Build history of the part. All positions in model axes, mm. A direction names the side the tool comes from. Give positions to 0.01 mm unless a question says otherwise; leave off trailing zeros. Write each loop counter-clockwise with the first axis right and the second up, starting at its lowest first coordinate (ties: lowest second). Pieces come first, ordered by that corner, then holes. Notation, with made-up numbers: (86, 6) -> (144, 6) arc R36 ccw to (144, 40) -> close; hole circle Ø11 at (5.5, 67). An arc over 180 degrees is marked (long way). Write item = value, one per line. Start each with the question number.
Q1. Wall check: line 1 (Y direction, x = 9.25, z = 0); line 2 (X direction, y = -1.5, z = -13); line 3 (Z direction, x = 1.5, y = 2). Give the ranges that are in metal, low to high.
Q2. Saw through at C-C, the plane x = 2.5. List the corners of the cut face in (y, z), then the cut area to 3 significant figures.
Q3. Mould opens along Y. For faces 1 (the face through (2.03, -3.47, 15.62)), 2 (the face through (15, 0, 3)), 3 (the face through (7.4, -2.26, 1.18)) say: pulls with the +Y half, pulls with the -Y half, needs draft (parallel to the pull), parting line crosses it, or undercut.
Q4. Tool access for faces 4 (the face through (0, 0, 3)), 5 (the face through (4, -10, 8)): list every direction of +Z, -Z, +X, -X, +Y, -Y with a clear straight run to the whole face (end or side of a thin tool).
Q5. Drop flat-ended pins along their axis: P1, Ø4, axis at x = 8, y = -4.5, coming from the -Z side; P2, Ø1.5, axis at x = 5, z = 3, coming from the -Y side; P3, Ø2, axis at y = 4.5, z = -2, coming from the -X side; P4, Ø2, axis at x = 4.5, z = -7, coming from the +Y side. Give the stop position or say it passes through.
Q6. Saw through at D-D, the plane y = -11. List the corners of the cut face in (x, z).
Q7. Saw through at A-A, the plane y = 0. List the corners of the cut face in (x, z), then the cut area to 4 significant figures.
from build123d import *

# Parameters (mm, degrees)
SKETCH2_R          = 2.55
CUT_EXTRUDE1_DEPTH = 15


with BuildPart() as part:
    # Sketch1 → Revolve1 (revolve)
    with BuildSketch(Plane.XY):
        Polygon((0, 0), (0, 16), (4, 16), (4, 12.5), (11, 12.5), (11, 16), (15, 16), (15, 0), align=None)
    revolve(axis=Axis((15, 0, 0), (-1, 0, 0)))

    # Sketch2 → Cut-Extrude1 (cut)
    with BuildSketch(Plane.ZY):
        Circle(SKETCH2_R)
    extrude(amount=-CUT_EXTRUDE1_DEPTH, mode=Mode.SUBTRACT)


solid = part.part
Report:
q1.line_1 = -12.5 to -2.55, 2.55 to 12.5
q1.line_2 = 0 to 4, 11 to 15
q1.line_3 = -15.87 to -1.58, 1.58 to 15.87
q2.outline = circle Ø32 at (0, 0); hole circle Ø5.1 at (0, 0)
q2.area = 784 mm2
q3.face_1 = parting line crosses it
q3.face_2 = needs draft
q3.face_3 = undercut
q4.face_4 = +Z, -Z, -X, +Y, -Y
q4.face_5 = none
q5.P1 = -12.25
q5.P2 = -12.3
q5.P3 = 0
q5.P4 = 14.78
q6.outline = (0, -11.62) -> (4, -11.62) -> (4, -5.94) -> (11, -5.94) -> (11, -11.62) -> (15, -11.62) -> (15, 11.62) -> (11, 11.62) -> (11, 5.94) -> (4, 5.94) -> (4, 11.62) -> (0, 11.62) -> close
q7.outline = (0, -16) -> (4, -16) -> (4, -12.5) -> (11, -12.5) -> (11, -16) -> (15, -16) -> (15, -2.55) -> (0, -2.55) -> close; (0, 2.55) -> (15, 2.55) -> (15, 16) -> (11, 16) -> (11, 12.5) -> (4, 12.5) -> (4, 16) -> (0, 16) -> close
q7.area = 354.5 mm2
